from build123d import *

# Parameters (mm, degrees)
F1_DEPTH = 10.16


with BuildPart() as f1:
    # F0 (on Top) → F1 (new body)
    with BuildSketch(Plane.XY):
        Polygon((31.75, 0), (19.05, 0), (19.05, -10.16), (0, -10.16), (0, -31.75), (10.16, -31.75), (10.16, -44.45), (0, -44.45), (0, -57.15), (10.16, -57.15), (10.16, -69.85), (0, -69.85), (0, -82.55), (10.16, -82.55), (10.16, -95.25), (0, -95.25), (0, -107.95), (10.16, -107.95), (10.16, -120.65), (0, -120.65), (0, -133.35), (10.16, -133.35), (10.16, -146.05), (0, -146.05), (0, -167.64), (19.05, -167.64), (19.05, -177.8), (31.75, -177.8), (31.75, -167.64), (44.45, -167.64), (44.45, -177.8), (57.15, -177.8), (57.15, -167.64), (69.85, -167.64), (69.85, -177.8), (82.55, -177.8), (82.55, -167.64), (95.25, -167.64), (95.25, -177.8), (107.95, -177.8), (107.95, -167.64), (120.65, -167.64), (120.65, -177.8), (133.35, -177.8), (133.35, -167.64), (146.05, -167.64), (146.05, -177.8), (158.75, -177.8), (158.75, -167.64), (171.45, -167.64), (171.45, -177.8), (184.15, -177.8), (184.15, -167.64), (196.85, -167.64), (196.85, -177.8), (209.55, -177.8), (209.55, -167.64), (228.6, -167.64), (228.6, -146.05), (218.44, -146.05), (218.44, -133.35), (228.6, -133.35), (228.6, -120.65), (218.44, -120.65), (218.44, -107.95), (228.6, -107.95), (228.6, -95.25), (218.44, -95.25), (218.44, -82.55), (228.6, -82.55), (228.6, -69.85), (218.44, -69.85), (218.44, -57.15), (228.6, -57.15), (228.6, -44.45), (218.44, -44.45), (218.44, -31.75), (228.6, -31.75), (228.6, -10.16), (209.55, -10.16), (209.55, 0), (196.85, 0), (196.85, -10.16), (184.15, -10.16), (184.15, 0), (171.45, 0), (171.45, -10.16), (158.75, -10.16), (158.75, 0), (146.05, 0), (146.05, -10.16), (133.35, -10.16), (133.35, 0), (120.65, 0), (120.65, -10.16), (107.95, -10.16), (107.95, 0), (95.25, 0), (95.25, -10.16), (82.55, -10.16), (82.55, 0), (69.85, 0), (69.85, -10.16), (57.15, -10.16), (57.15, 0), (44.45, 0), (44.45, -10.16), (31.75, -10.16), align=None)
    extrude(amount=F1_DEPTH)


solid = f1.part
The listing builds one solid part. Answer for the finished solid, in the listing's coordinates (mm). A direction names the side the tool comes from. Coordinates: 2 decimals unless noted, no trailing zeros. Order: outer loops, then holes, each group sorted by start corner. A loop starts at its lowest first (then second) coordinate and runs counter-clockwise, first axis right, second up. Notation, with made-up numbers: (-38.75, 40) -> (-8.75, 40) arc R10 ccw to (-8.75, 46) -> close; hole circle Ø7 at (52, 39). An arc over 180 degrees is marked (long way). Answer in a Markdown table with one row per item. Add a question column.
Item 1: Find section B-B (x = 113). Write down the section's boundary in (y, z), then the cut area to 3 significant figures.
Item 2: Which of the six approach directions +Z, -Z, +X, -X, +Y, -Y give full straight-line access (tool end or side, diameter ignored) to faces 4 (the face through (10.16, -63, 5)), 5 (the face through (178, 0, 5)), 6 (the face through (165, -167.64, 5)), 7 (the face through (69.85, -5, 5)), 8 (the face through (10, -10.16, 5))?
Item 3: Find the intervals of material crossed by L1, parallel to Y at x = 193, z = 5.5; L2, parallel to X at y = -36, z = 7.5, in increasing order. Write a range as from..to.
Item 4: Each of these flat-tipped pins is pushed along its axis until it touches: P1, Ø3, axis at y = -5.5, z = 2.5, coming from the +X side; P2, Ø5, axis at y = -61.5, z = 2.5, coming from the -X side; P3, Ø5, axis at y = -171.5, z = 4.5, coming from the -X side. Where does it stop, or does it pass through?
Item 5: Find section A-A (y = -112). Write down the section's boundary in (x, z), then the cut area to 3 significant figures.
Item 6: Determine the mould class of faces 1 (the face through (69.85, -173, 5)), 2 (the face through (219, -10.16, 5)), 3 (the face through (224, -44.45, 5)) for opening direction Y: +Y half, -Y half, draft (parallel to the pull), parting line (faces both ways), or undercut.
Result set:
| question | item | result |
|---|---|---|
| 1 | outline | (-167.64, 0) -> (-10.16, 0) -> (-10.16, 10.16) -> (-167.64, 10.16) -> close |
| 1 | area | 1,600 mm² |
| 2 | face 4 | +Z, -Z, -X |
| 2 | face 5 | +Z, -Z, +X, -X, +Y |
| 2 | face 6 | +Z, -Z, -Y |
| 2 | face 7 | +Z, -Z, +Y |
| 2 | face 8 | +Z, -Z, -X, +Y |
| 3 | L1 | y = -167.64..-10.16 |
| 3 | L2 | x = 10.16..218.44 |
| 4 | P1 | stops at x = 209.55 |
| 4 | P2 | stops at x = 10.16 |
| 4 | P3 | stops at x = 19.05 |
| 5 | outline | (10.16, 0) -> (218.44, 0) -> (218.44, 10.16) -> (10.16, 10.16) -> close |
| 5 | area | 2,120 mm² |
| 6 | face 1 | draft |
| 6 | face 2 | +Y half |
| 6 | face 3 | undercut |
